Geometry: final body of the model. Coordinates: model frame, mm. Face numbers are marked on the shaded views. A direction names the side the tool comes from. Coordinates: 2 decimals unless noted, no trailing zeros. Loops run counter-clockwise (first coordinate to the right, second up) from the corner with the lowest first, then second, coordinate; pieces in that order, holes last. Notation, with made-up numbers: (-39, -11) - (-3, -11) arc R16 cw to (-3, -4) - close; hole circle Ø1 at (-13, 38). An arc over 180 degrees is marked (long way). Return JSON: item names as keys, results as strings.
from build123d import *

# Parameters (mm, degrees)
EXTRUDE_1_DEPTH     = 30
SKETCH_3_R          = 2
CUT_EXTRUDE_2_DEPTH = 10
SKETCH_4_R          = 2
CUT_EXTRUDE_3_DEPTH = 10
SKETCH_2_R          = 1.8
CUT_EXTRUDE_4_DEPTH = 20
SKETCH_5_W          = 8
SKETCH_5_H          = 7.5
CUT_EXTRUDE_5_DEPTH = 30
SKETCH_6_R          = 2
CUT_EXTRUDE_6_DEPTH = 10


with BuildPart() as part:
    # 草圖1 → 填料-伸長1 (new body)
    with BuildSketch(Plane(origin=(0, 0, 0), x_dir=(1, 0, 0), z_dir=(0, 1, 0))):
        Polygon((0, 0), (0, 107.1), (80.5, 107.1), (80.5, 102.1), (8, 102.1), (8, 0), align=None)
    extrude(amount=EXTRUDE_1_DEPTH)

    # 草圖3 → 除料-伸長2 (cut)
    with BuildSketch(Plane.ZY):
        with Locations((-25, 23)):
            Circle(SKETCH_3_R)
        with Locations((-25, 15)):
            Circle(SKETCH_3_R)
        with Locations((-25, 7)):
            Circle(SKETCH_3_R)
        with Locations((-33, 23)):
            Circle(SKETCH_3_R)
        with Locations((-33, 15)):
            Circle(SKETCH_3_R)
        with Locations((-33, 7)):
            Circle(SKETCH_3_R)
        with Locations((-63.1, 23)):
            Circle(SKETCH_3_R)
        with Locations((-64.092277877, 15.061776986)):
            Circle(SKETCH_3_R)
        with Locations((-64.099940822, 7.061780656)):
            Circle(SKETCH_3_R)
        with Locations((-71.1, 23)):
            Circle(SKETCH_3_R)
        with Locations((-72.092277877, 15.061776986)):
            Circle(SKETCH_3_R)
        with Locations((-72.099940822, 7.061780656)):
            Circle(SKETCH_3_R)
        with Locations((-79.1, 23)):
            Circle(SKETCH_3_R)
        with Locations((-80.092277877, 15.061776986)):
            Circle(SKETCH_3_R)
        with Locations((-80.099940822, 7.061780656)):
            Circle(SKETCH_3_R)
        with Locations((-87.1, 23)):
            Circle(SKETCH_3_R)
        with Locations((-88.092277877, 15.061776986)):
            Circle(SKETCH_3_R)
        with Locations((-88.099940822, 7.061780656)):
            Circle(SKETCH_3_R)
    extrude(amount=-CUT_EXTRUDE_2_DEPTH, mode=Mode.SUBTRACT)

    # 草圖4 → 除料-伸長3 (cut)
    with BuildSketch(Plane(origin=(0, 0, -107.1), x_dir=(-1, 0, 0), z_dir=(0, 0, -1))):
        with Locations((-74.2, 26)):
            Circle(SKETCH_4_R)
        with Locations((-74.2, 18)):
            Circle(SKETCH_4_R)
        with Locations((-74.2, 10)):
            Circle(SKETCH_4_R)
    extrude(amount=-CUT_EXTRUDE_3_DEPTH, mode=Mode.SUBTRACT)

    # 草圖2 → 除料-伸長4 (cut)
    with BuildSketch(Plane.XY):
        with Locations((4, 23)):
            Circle(SKETCH_2_R)
        with Locations((4, 7)):
            Circle(SKETCH_2_R)
        with Locations((4, 15)):
            Circle(SKETCH_2_R)
    extrude(amount=-CUT_EXTRUDE_4_DEPTH, mode=Mode.SUBTRACT)

    # 草圖5 → 除料-伸長5 (cut)
    with BuildSketch(Plane(origin=(0, 30, 0), x_dir=(1, 0, 0), z_dir=(0, 1, 0))):
        with Locations((4, 3.75)):
            Rectangle(SKETCH_5_W, SKETCH_5_H)
    extrude(amount=-CUT_EXTRUDE_5_DEPTH, mode=Mode.SUBTRACT)

    # 草圖6 → 除料-伸長6 (cut)
    with BuildSketch(Plane(origin=(0, 0, -107.1), x_dir=(-1, 0, 0), z_dir=(0, 0, -1))):
        with Locations((-56.067683871, 27)):
            Circle(SKETCH_6_R)
        with Locations((-56.067683871, 19)):
            Circle(SKETCH_6_R)
        with Locations((-56.067683871, 11)):
            Circle(SKETCH_6_R)
        with Locations((-32.067683871, 27)):
            Circle(SKETCH_6_R)
        with Locations((-32.067683871, 19)):
            Circle(SKETCH_6_R)
        with Locations((-32.067683871, 11)):
            Circle(SKETCH_6_R)
        with Locations((-56.067683871, 3)):
            Circle(SKETCH_6_R)
        with Locations((-32.067683871, 3)):
            Circle(SKETCH_6_R)
    extrude(amount=-CUT_EXTRUDE_6_DEPTH, mode=Mode.SUBTRACT)


solid = part.part
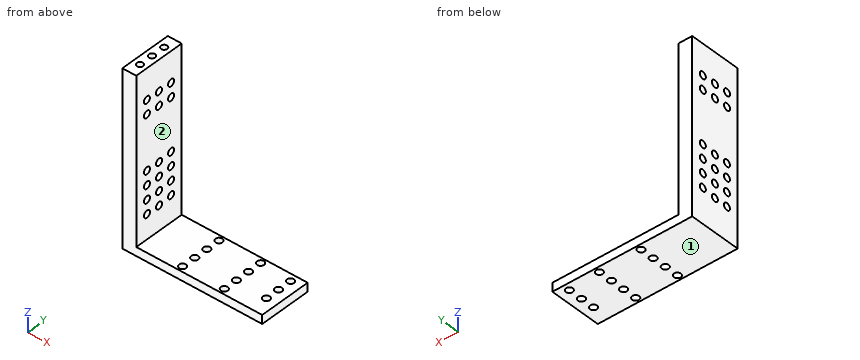
Item 1: Section query B-B, the plane z = -25. Return loops of the section in (x, y).
Worked out:
{"outline": "(0, 0) - (8, 0) - (8, 5) - (0, 5) - close; (0, 9) - (8, 9) - (8, 13) - (0, 13) - close; (0, 17) - (8, 17) - (8, 21) - (0, 21) - close; (0, 25) - (8, 25) - (8, 30) - (0, 30) - close"}
Item 2: Reachability of the marked faces 1 and 2 from +Z, -Z, +X, -X, +Y, -Y: full face, straight path, thin tool, end or side. Return the list, or none.
Worked out:
{"face 1": "-Z, +X, -X, +Y, -Y", "face 2": "+Z, +X, +Y, -Y"}
Item 3: Section query D-D, the plane z = -97. Return loops of the section in (x, y), and give its area (3 significant figures).
Worked out:
{"outline": "(0, 0) - (8, 0) - (8, 30) - (0, 30) - close", "area": "240 mm^2"}
Item 4: Ray query, probe 1 along Y at (x, z) = (6, -25); probe 2 along Y at (x, z) = (74.2, -105.95); probe 3 along Z at (x, y) = (40, 25). Return the intervals inside material, ascending. Write a range as from..to.
Worked out:
{"probe 1": "0..5, 9..13, 17..21, 25..30", "probe 2": "0..8, 12..16, 20..24, 28..30", "probe 3": "-107.1..-102.1"}
Item 5: Section query C-C, the plane x = 4. Count the separate pieces of the cut face and the enclosed holes in it, and give its area (3 significant figures).
Worked out:
{"separate pieces": "1", "enclosed holes": "18", "area": "2,630 mm^2"}
Item 6: Section query A-A, the plane x = 74.2. Return loops of the section in (y, z), and give its area (3 significant figures).
Worked out:
{"outline": "(0, -107.1) - (8, -107.1) - (8, -102.1) - (0, -102.1) - close; (12, -107.1) - (16, -107.1) - (16, -102.1) - (12, -102.1) - close; (20, -107.1) - (24, -107.1) - (24, -102.1) - (20, -102.1) - close; (28, -107.1) - (30, -107.1) - (30, -102.1) - (28, -102.1) - close", "area": "90.0 mm^2"}
Item 7: First-contact query: pin 1 Ø3.5 at (x, y) = (74.2, 10) entering from +Z; pin 2 Ø2 at (y, z) = (19.5, -68) entering from +X; pin 3 Ø3 at (x, y) = (64, 25) entering from +Z. Flat tips, straight axial feed; report the tip coordinate or a pass-through.
Worked out:
{"pin 1": "through", "pin 2": "x = 8", "pin 3": "z = -102.1"}
